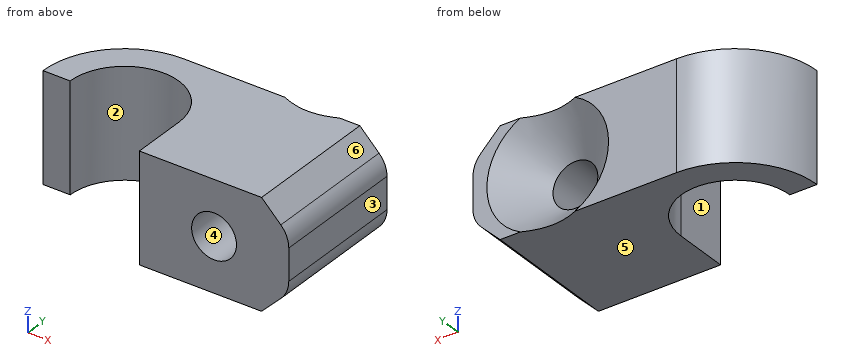
from build123d import *

# Parameters (mm, degrees)
F1_DEPTH       = 4
F3_D           = 3.3
F3_CSINK_D     = 8.96
F3_CSINK_ANGLE = 90
F4_SIZE        = 2
F5_R           = 2


with BuildPart() as f1:
    # F0 (on Top) → F1 (new body, symmetric)
    with BuildSketch(Plane.XY):
        with BuildLine():
            ThreePointArc((-4, 0), (0, 4), (4, 0))
            Line((4, 0), (4, -4.0273182094))
            Line((4, -4.0273182094), (15, -4.0273182094))
            Line((15, -4.0273182094), (15, 6))
            Line((15, 6), (0, 6))
            ThreePointArc((0, 6), (-4.2426406871, 4.2426406871), (-6, 0))
            Line((-6, 0), (-4, 0))
        make_face()
    extrude(amount=F1_DEPTH, both=True)

    # F3 (through all)
    with Locations(Plane(origin=(0, 6, 0), x_dir=(-1, 0, 0), z_dir=(0, 1, 0))):
        with Locations((-9.5, 0)):
            CounterSinkHole(F3_D / 2, F3_CSINK_D / 2, counter_sink_angle=F3_CSINK_ANGLE)

    # F4
    f4_edges = [f1.edges().sort_by_distance(p)[0] for p in [
        (15, 0.986341, -4),
        (15, 0.986341, 4),
    ]]
    chamfer(f4_edges, length=F4_SIZE)

    # F5
    f5_edges = [f1.edges().sort_by_distance(p)[0] for p in [
        (15, 0.986341, -2),
        (15, 0.986341, 2),
    ]]
    fillet(f5_edges, radius=F5_R)


solid = f1.part
Can you work these out from the model? Positions are in its coordinate system, mm. Face numbers are marked on the shaded views. A direction names the side the tool comes from. Give positions to 0.01 mm unless a question says otherwise; leave off trailing zeros. Write each loop counter-clockwise with the first axis right and the second up, starting at its lowest first coordinate (ties: lowest second). Pieces come first, ordered by that corner, then holes. Notation, with made-up numbers: (8, 67.5) -> (45, 67.5) arc R23 cw to (45, 94.5) -> close; hole circle Ø8 at (51.25, -28). An arc over 180 degrees is marked (long way). Answer as a JSON object with one key per item and string values. Group by question number.
Item 1: Please list where these lines run through material, in increasing order: line 1 (X direction, y = -0.25, z = 0); line 2 (X direction, y = 1.5, z = 0); line 3 (Z direction, x = 9.5, y = -0.5). Write a range as [from, to].
Item 2: Suppose I cut it at D-D (y = -2). Please give me the cut outline in (x, z), plus the area to 3 significant figures.
Item 3: Suppose I cut it at A-A (x = 9.5). Please give me the cut outline in (y, z), plus the area to 4 significant figures.
Item 4: Suppose I cut it at B-B (z = 0). Please give me the cut outline in (x, y), plus the area to 3 significant figures.
Item 5: Suppose I cut it at C-C (y = 3.5). Please give me the cut outline in (x, z).
Item 6: I'm going to push flat-ended pins straight in: P1, Ø1.5, axis at x = -4, z = -1.5, coming from the +Y side; P2, Ø6, axis at x = -4, y = 4.5, coming from the +Z side; P3, Ø1.5, axis at x = 2.5, z = 1.5, coming from the -Y side; P4, Ø2, axis at x = -5, z = 1, coming from the -Y side. Where does each tip first touch, or does it pass through?
Item 7: We'd pull the mould along Z, two halves only. Please class the marked faces 3, 4, 5 and 6: +Z half, -Z half, draft (parallel to the pull), parting line (faces both ways), or undercut.
Item 8: For the marked faces 1 and 2, which set-ups out of +Z, -Z, +X, -X, +Y, -Y let a thin tool reach every point of the face, with its end or its side?
Findings:
{
 "1": {"line 1": "x = [4, 7.85], [11.15, 15]", "line 2": "x = [-5.81, -3.71], [3.71, 7.85], [11.15, 15]", "line 3": "z = [-4, -1.65], [1.65, 4]"},
 "2": {"outline": "(4, -4) -> (13, -4) -> (14.41, -2.59) arc R2 ccw to (15, -1.17) -> (15, 1.17) arc R2 ccw to (14.41, 2.59) -> (13, 4) -> (4, 4) -> close; hole circle Ø3.3 at (9.5, 0)", "area": "75.3 mm²"},
 "3": {"outline": "(-4.03, -4) -> (5.52, -4) -> (3.17, -1.65) -> (-4.03, -1.65) -> close; (-4.03, 1.65) -> (3.17, 1.65) -> (5.52, 4) -> (-4.03, 4) -> close", "area": "39.35 mm²"},
 "4": {"outline": "(-6, 0) -> (-4, 0) arc R4 cw to (4, 0) -> (4, -4.03) -> (7.85, -4.03) -> (7.85, 3.17) -> (5.02, 6) -> (0, 6) arc R6 ccw to start; (11.15, -4.03) -> (15, -4.03) -> (15, 6) -> (13.98, 6) -> (11.15, 3.17) -> close", "area": "96.3 mm²"},
 "5": {"outline": "(-4.87, -4) -> (-1.94, -4) -> (-1.94, 4) -> (-4.87, 4) -> close; (1.94, -4) -> (13, -4) -> (14.41, -2.59) arc R2 ccw to (15, -1.17) -> (15, 1.17) arc R2 ccw to (14.41, 2.59) -> (13, 4) -> (1.94, 4) -> close; hole circle Ø3.96 at (9.5, 0)"},
 "6": {"P1": "stops at y = 5.04", "P2": "stops at z = 4", "P3": "stops at y = 2.33", "P4": "stops at y = 0"},
 "7": {"face 3": "draft", "face 4": "undercut", "face 5": "-Z half", "face 6": "+Z half"},
 "8": {"face 1": "+Z, -Z, -X, -Y", "face 2": "+Z, -Z, -Y"}
}
